from build123d import *

# Parameters (mm, degrees)
F1_DEPTH = 1.5


with BuildPart() as f1:
    # F0 (on Top) → F1 (new body)
    with BuildSketch(Plane.XY):
        with BuildLine():
            Line((-7.893, 4), (-9.5, 4))
            Line((-9.5, 4), (-9.5, -4))
            Line((-9.5, -4), (9.5, -4))
            Line((9.5, -4), (9.5, 4))
            Line((9.5, 4), (7.893, 4))
            Line((7.893, 4), (7.893, 3.6))
            ThreePointArc((7.893, 3.6), (7.493, 3.2), (7.093, 3.6))
            Line((7.093, 3.6), (7.093, 4))
            Line((7.093, 4), (6.3944, 4))
            Line((6.3944, 4), (6.3944, 3.6))
            ThreePointArc((6.3944, 3.6), (5.9944, 3.2), (5.5944, 3.6))
            Line((5.5944, 3.6), (5.5944, 4))
            Line((5.5944, 4), (4.8958, 4))
            Line((4.8958, 4), (4.8958, 3.6))
            ThreePointArc((4.8958, 3.6), (4.4958, 3.2), (4.0958, 3.6))
            Line((4.0958, 3.6), (4.0958, 4))
            Line((4.0958, 4), (3.3972, 4))
            Line((3.3972, 4), (3.3972, 3.6))
            ThreePointArc((3.3972, 3.6), (2.9972, 3.2), (2.5972, 3.6))
            Line((2.5972, 3.6), (2.5972, 4))
            Line((2.5972, 4), (1.8986, 4))
            Line((1.8986, 4), (1.8986, 3.6))
            ThreePointArc((1.8986, 3.6), (1.4986, 3.2), (1.0986, 3.6))
            Line((1.0986, 3.6), (1.0986, 4))
            Line((1.0986, 4), (0.4, 4))
            Line((0.4, 4), (0.4, 3.6))
            ThreePointArc((0.4, 3.6), (0, 3.2), (-0.4, 3.6))
            Line((-0.4, 3.6), (-0.4, 4))
            Line((-0.4, 4), (-1.0986, 4))
            Line((-1.0986, 4), (-1.0986, 3.6))
            ThreePointArc((-1.0986, 3.6), (-1.4986, 3.2), (-1.8986, 3.6))
            Line((-1.8986, 3.6), (-1.8986, 4))
            Line((-1.8986, 4), (-2.5972, 4))
            Line((-2.5972, 4), (-2.5972, 3.6))
            ThreePointArc((-2.5972, 3.6), (-2.9972, 3.2), (-3.3972, 3.6))
            Line((-3.3972, 3.6), (-3.3972, 4))
            Line((-3.3972, 4), (-4.0958, 4))
            Line((-4.0958, 4), (-4.0958, 3.6))
            ThreePointArc((-4.0958, 3.6), (-4.4958, 3.2), (-4.8958, 3.6))
            Line((-4.8958, 3.6), (-4.8958, 4))
            Line((-4.8958, 4), (-5.5944, 4))
            Line((-5.5944, 4), (-5.5944, 3.6))
            ThreePointArc((-5.5944, 3.6), (-5.9944, 3.2), (-6.3944, 3.6))
            Line((-6.3944, 3.6), (-6.3944, 4))
            Line((-6.3944, 4), (-7.093, 4))
            Line((-7.093, 4), (-7.093, 3.6))
            ThreePointArc((-7.093, 3.6), (-7.493, 3.2), (-7.893, 3.6))
            Line((-7.893, 3.6), (-7.893, 4))
        make_face()
    extrude(amount=F1_DEPTH)


solid = f1.part
The model under review builds one solid part; all positions refer to its coordinate system, in mm. Round coordinates to 2 decimals unless told otherwise and drop trailing zeros. Loops run counter-clockwise (first coordinate to the right, second up) from the corner with the lowest first, then second, coordinate; pieces in that order, holes last. Notation, with made-up numbers: (32.5, -37) -> (85.5, -37) arc R20 cw to (85.5, -33) -> close; hole circle Ø2 at (1.25, 75.5). An arc over 180 degrees is marked (long way). One line per question, with ' | ' between items. Start each with the question number.
Item 1: Wall thickness on line 1 along Y through (x, z) = (7.5, 0.2); line 2 along Y through (x, z) = (1.25, 0.45): over which ranges is each line inside the solid? List them lowest first. Write a range as [from, to].
Item 2: Add section A-A, the plane x = 0. Write out the cut boundary in (y, z).
Item 3: Draft analysis for pull direction X (two halves, no side actions). For faces 1 (the face through (-9, 4, 1)), 2 (the face through (9.5, 0, 1)), 3 (the face through (-6, 3.2, 0.7)), state which applies: +X half, -X half, draft (parallel to the pull), parting line (faces both ways), or undercut.
Return value:
1) line 1: y = [-4, 3.2] | line 2: y = [-4, 3.29]
2) outline: (-4, 0) -> (3.2, 0) -> (3.2, 1.5) -> (-4, 1.5) -> close
3) face 1: draft | face 2: +X half | face 3: undercut
